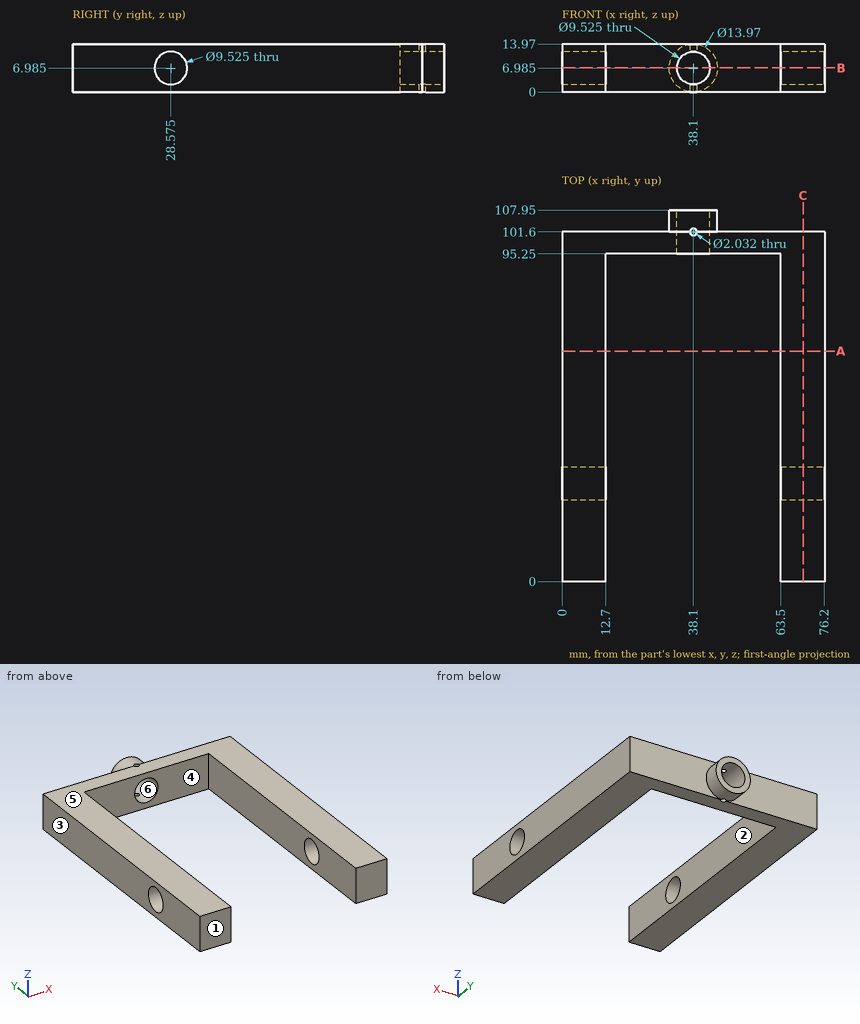
Part print with two shaded views. Sizes in mm from the minimum x, y, z corner. A direction names the side the tool comes from. Coordinates: 2 decimals unless noted, no trailing zeros. Write each loop counter-clockwise with the first axis right and the second up, starting at its lowest first coordinate (ties: lowest second). Pieces come first, ordered by that corner, then holes.
(1) Cut at A-A on y = 67. List the corners of the cut face in (x, z), and give its area (3 significant figures).
(2) 3-axis set-ups, long thin cutter, end or side, ignore diameter. For the marked faces 1 and 2: which of +Z, -Z, +X, -X, +Y, -Y reach the whole face in a straight line?
(3) Cut at B-B on z = 7. List the corners of the cut face in (x, y).
(4) Pin check, flat tip, straight feed: pin 1 Ø4 at (x, z) = (27.5, 8.5) entering from +Y. Stop position of the tip, or through.
(5) Cut at C-C on x = 70. List the corners of the cut face in (y, z) (1 decimal).
(6) Mould opens along X. For the marked faces 3, 4, 5 and 6 say: pulls with the +X half, pulls with the -X half, needs draft (parallel to the pull), parting line crosses it, or undercut.
(7) Drill centre lines: line 1 (X direction, y = 19, z = 11.5); line 2 (Y direction, x = 50.5, z = 11.75); line 3 (Y direction, x = 67, z = 1.5). Where is each one in solid material? Low to high.
Working result:
1. outline: (0, 0) - (12.7, 0) - (12.7, 13.97) - (0, 13.97) - close; (63.5, 0) - (76.2, 0) - (76.2, 13.97) - (63.5, 13.97) - close
1. area: 355 mm2
2. face 1: +Z, -Z, +X, -X, -Y
2. face 2: +Z, -Z, -Y
3. outline: (0, 0) - (12.7, 0) - (12.7, 23.81) - (0, 23.81) - close; (0, 33.34) - (12.7, 33.34) - (12.7, 95.25) - (33.34, 95.25) - (33.34, 107.95) - (31.12, 107.95) - (31.12, 101.6) - (0, 101.6) - close; (42.86, 95.25) - (63.5, 95.25) - (63.5, 33.34) - (76.2, 33.34) - (76.2, 101.6) - (45.08, 101.6) - (45.08, 107.95) - (42.86, 107.95) - close; (63.5, 0) - (76.2, 0) - (76.2, 23.81) - (63.5, 23.81) - close
4. pin 1: stops at y = 101.6
5. outline: (0, 0) - (101.6, 0) - (101.6, 14) - (0, 14) - close; hole circle Ø9.5 at (28.6, 7)
6. face 3: pulls with the -X half
6. face 4: undercut
6. face 5: needs draft
6. face 6: undercut
7. line 1: x = 0 to 12.7, 63.5 to 76.2
7. line 2: y = 95.25 to 101.6
7. line 3: y = 0 to 101.6
